Input: part model. Units: mm. Frame: model coordinates. Face numbers are marked on the shaded views. A direction names the side the tool comes from. Coordinates: 2 decimals unless noted, no trailing zeros. Write each loop counter-clockwise with the first axis right and the second up, starting at its lowest first coordinate (ties: lowest second). Pieces come first, ordered by that corner, then holes. Notation, with made-up numbers: M 39.5,9 L 54.5,9 A26 ccw 54.5,37 Z; hole C 52,3 d4. An arc over 180 degrees is marked long. Write each question's results on one line, items separated by ' | '. Start each with the question number.
1. Section query C-C, the plane y = -20. Output: boundary loops of the cut face in (x, z), and give its area (3 significant figures).
2. Section query B-B, the plane y = -17. Output: boundary loops of the cut face in (x, z), and give its area (3 significant figures).
3. Ray query, probe 1 along Z at (x, y) = (-32.75, -23.75); probe 2 along Y at (x, z) = (-36, -22.8); probe 3 along Y at (x, z) = (-27, -0.15). Return the intervals inside material, ascending.
4. First-contact query: pin 1 (1.5 mm diameter, centred on x = -40.5, z = -17.5, fed in from -Y); pin 2 (3.5 mm diameter, centred on y = -21, z = -15.5, fed in from +X); pin 3 (2 mm diameter, centred on x = -28, y = -23, fed in from -Z); pin 4 (6 mm diameter, centred on x = -25, y = -24.5, fed in from -Z). Flat tips, straight axial feed; report the tip coordinate or a pass-through.
5. Section query A-A, the plane x = -36. Output: boundary loops of the cut face in (y, z).
6. Set-up query: the marked faces 4 and 5. Return all of +Z, -Z, +X, -X, +Y, -Y with unobstructed straight access to the full face (end or side cutting, diameter ignored); none if empty.
7. Section query D-D, the plane z = -6. Output: boundary loops of the cut face in (x, y), and give its area (3 significant figures).
8. Pull-direction query (Y, two-part tool) for the marked faces 1, 2 and 3; classes: +Y half, -Y half, draft (parallel to the pull), parting line (faces both ways), or undercut.
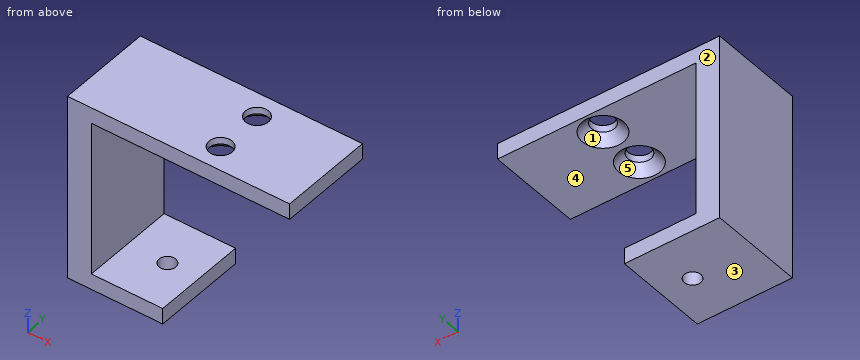
```python
from build123d import *

# Parameters (mm, degrees)
LINK_EYE_SHELF_START          = -23.5
SKETCH1_W                     = 12
SKETCH1_H                     = 12
SKETCH1_R                     = 1.05
LINK_EYE_SHELF_DEPTH          = 2
OUTBOARD_WEB_START            = -22.5
SKETCH2_W                     = 3
SKETCH2_H                     = 12
OUTBOARD_WEB_DEPTH            = 21.5
CARRIAGE_PLATE_FOOT_START     = -2
SKETCH3_W                     = 28
SKETCH3_H                     = 12
CARRIAGE_PLATE_FOOT_DEPTH     = 2
SKETCH6_R                     = 1.45
YTAB_D2P9_DEPTH               = 2.01
SKETCH7_R                     = 2.6
YTAB_CSK_D5P2_DEPTH           = 1.15
YTAB_CSK_D5P2_DRAFT           = -45
YTAB_CSK_D5P2_PROFILE_2_DEPTH = 1.15
YTAB_CSK_D5P2_PROFILE_2_DRAFT = -45


with BuildPart() as part:
    # Sketch1 → Link_Eye_Shelf (new body)
    with BuildSketch(Plane.XY.offset(LINK_EYE_SHELF_START)):
        with Locations((-38, -20)):
            Rectangle(SKETCH1_W, SKETCH1_H)
        with Locations((-36, -20)):
            Circle(SKETCH1_R, mode=Mode.SUBTRACT)
    extrude(amount=LINK_EYE_SHELF_DEPTH)

    # Sketch2 → Outboard_Web (add)
    with BuildSketch(Plane.XY.offset(OUTBOARD_WEB_START)):
        with Locations((-42.5, -20)):
            Rectangle(SKETCH2_W, SKETCH2_H)
    extrude(amount=OUTBOARD_WEB_DEPTH)

    # Sketch3 → Carriage_Plate_Foot (add)
    with BuildSketch(Plane.XY.offset(CARRIAGE_PLATE_FOOT_START)):
        with Locations((-30, -20)):
            Rectangle(SKETCH3_W, SKETCH3_H)
    extrude(amount=CARRIAGE_PLATE_FOOT_DEPTH)

    # Sketch6 → YTab_D2p9 (cut)
    with BuildSketch(Plane(origin=(0, 0, -2), x_dir=(-1, 0, 0), z_dir=(0, 0, -1))):
        with Locations((27, -23)):
            Circle(SKETCH6_R)
        with Locations((27, -17)):
            Circle(SKETCH6_R)
    extrude(amount=-YTAB_D2P9_DEPTH, mode=Mode.SUBTRACT)


with BuildPart() as ytab_csk_d5p2_tool:
    # Sketch7 → YTab_CSK_D5p2 (with draft: the straight prism first)
    with BuildSketch(Plane(origin=(0, 0, -2), x_dir=(-1, 0, 0), z_dir=(0, 0, -1))):
        with Locations((27, -23)):
            Circle(SKETCH7_R)
    extrude(amount=-YTAB_CSK_D5P2_DEPTH)
    # YTab_CSK_D5p2: the draft: its side faces are tilted about the plane it starts from
    ytab_csk_d5p2_sides = [ytab_csk_d5p2_tool.faces().sort_by_distance(p)[0] for p in [
        (-24.4, -23, -1.425),
    ]]
    draft(ytab_csk_d5p2_sides, Plane(origin=(0, 0, -2), x_dir=(-1, 0, 0), z_dir=(0, 0, -1)), YTAB_CSK_D5P2_DRAFT)


with BuildPart() as part_1:
    add(part.part)

    # YTab_CSK_D5p2: cut by ytab_csk_d5p2_tool
    add(ytab_csk_d5p2_tool.part, mode=Mode.SUBTRACT)


with BuildPart() as ytab_csk_d5p2_profile_2_tool:
    # Sketch7 → YTab_CSK_D5p2 profile 2 (with draft: the straight prism first)
    with BuildSketch(Plane(origin=(0, 0, -2), x_dir=(-1, 0, 0), z_dir=(0, 0, -1))):
        with Locations((27, -17)):
            Circle(SKETCH7_R)
    extrude(amount=-YTAB_CSK_D5P2_PROFILE_2_DEPTH)
    # YTab_CSK_D5p2 profile 2: the draft: its side faces are tilted about the plane it starts from
    ytab_csk_d5p2_profile_2_sides = [ytab_csk_d5p2_profile_2_tool.faces().sort_by_distance(p)[0] for p in [
        (-24.4, -17, -1.425),
    ]]
    draft(ytab_csk_d5p2_profile_2_sides, Plane(origin=(0, 0, -2), x_dir=(-1, 0, 0), z_dir=(0, 0, -1)), YTAB_CSK_D5P2_PROFILE_2_DRAFT)


with BuildPart() as part_2:
    add(part_1.part)

    # YTab_CSK_D5p2 profile 2: cut by ytab_csk_d5p2_profile_2_tool
    add(ytab_csk_d5p2_profile_2_tool.part, mode=Mode.SUBTRACT)


solid = part_2.part
```
Answer:
1) outline: M -44,-23.5 L -37.05,-23.5 L -37.05,-21.5 L -41,-21.5 L -41,-2 L -16,-2 L -16,0 L -44,0 Z; M -34.95,-23.5 L -32,-23.5 L -32,-21.5 L -34.95,-21.5 Z | area: 134 mm^2
2) outline: M -44,-23.5 L -32,-23.5 L -32,-21.5 L -41,-21.5 L -41,-2 L -29.6,-2 L -28.45,-0.85 L -28.45,0 L -44,0 Z; M -25.55,-0.85 L -24.4,-2 L -16,-2 L -16,0 L -25.55,0 Z | area: 131 mm^2
3) probe 1: -23.5 to -21.5, -2 to 0 | probe 2: -26 to -21.05, -18.95 to -14 | probe 3: -26 to -24.45, -21.55 to -18.45, -15.55 to -14
4) pin 1: y = -26 | pin 2: x = -41 | pin 3: z = -1.4 | pin 4: z = -2
5) outline: M -26,-23.5 L -21.05,-23.5 L -21.05,-21.5 L -26,-21.5 Z; M -26,-2 L -14,-2 L -14,0 L -26,0 Z; M -18.95,-23.5 L -14,-23.5 L -14,-21.5 L -18.95,-21.5 Z
6) face 4: +X, +Y, -Y | face 5: -Z
7) outline: M -44,-26 L -41,-26 L -41,-14 L -44,-14 Z | area: 36.0 mm^2
8) face 1: undercut | face 2: +Y half | face 3: draft
